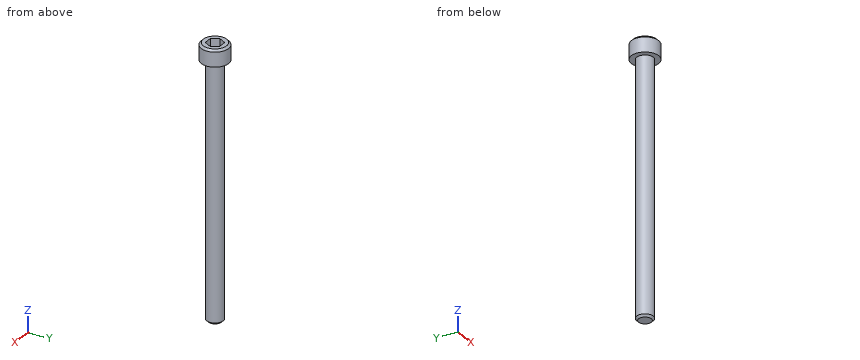
Autodesk Inventor part; units mm, degrees
ref_plane "YZ Plane" through (0, 0, 0) normal (1, 0, 0) x (0, 1, 0)
ref_plane "XZ Plane" through (0, 0, 0) normal (0, 1, 0) x (-1, 0, 0)
ref_plane "XY Plane" through (0, 0, 0) normal (0, 0, 1) x (1, 0, 0)
sketch "Sketch1" plane through (0, 0, 0) normal (0, 0, 1) x (1, 0, 0)
  circle A0 centre (0, 0) radius 3.429
  dimension "d0" = 6.858
extrude "Extrusion1" add sketch "Sketch1" along normal blind 4.1656
sketch "Sketch2" plane through (0, 0, 0) normal (0, 0, -1) x (-1, 0, 0)
  circle A0 centre (0, 0) radius 3.429
  circle A1 centre (0, 0) radius 2.0828
  dimension "d3" = 4.1656
extrude "Extrusion2" add sketch "Sketch2" along normal blind 63.5 contours A1
sketch "Sketch3" plane through (0, 0, 4.1656) normal (0, 0, 1) x (1, 0, 0)
  circle A0 centre (0, 0) radius 3.429
  line L0 (-1.0311, 1.7859) -> (1.0311, 1.7859)
  line L1 (1.0311, 1.7859) -> (2.0622, 0)
  line L2 (2.0622, 0) -> (1.0311, -1.7859)
  line L3 (1.0311, -1.7859) -> (-1.0311, -1.7859)
  line L4 (-1.0311, -1.7859) -> (-2.0622, 0)
  line L5 (-2.0622, 0) -> (-1.0311, 1.7859)
  dimension "d6" = 3.5719
extrude "Extrusion3" cut sketch "Sketch3" against normal blind 2.032 contours L0 L1 L2 L3 L4 L5
thread "Thread1"
chamfer "Chamfer1" distance 0.508 angle 45 1 edges at (2.0828, 0, -63.5)
chamfer "Chamfer2" distance 0.508 angle 45 1 edges at (-3.429, 0, 4.1656)
properties part number "10-32 x1000" material "Steel"
Geometry check sheet. Reference: the model listing, model coordinates, mm. Coordinates: 2 decimals unless noted, no trailing zeros. Order: outer loops, then holes, each group sorted by start corner. A loop starts at its lowest first (then second) coordinate and runs counter-clockwise, first axis right, second up. Notation, with made-up numbers: M 64,37 L 85,37 A32 ccw 85,70 Z; hole C 52,-5 d1. An arc over 180 degrees is marked long. One line per question, with ' | ' between items. Start each with the question number.
Item 1: Cross-section at B-B on z = -40.5. Enter the section's corners in (x, y).
Item 2: Gauge pin test, flat ends, axial feed: pin 1 (1 mm diameter, centred on y = 2, z = -54, fed in from -X) (3 decimals); pin 2 (3 mm diameter, centred on x = -2, z = -9, fed in from +Y); pin 3 (2 mm diameter, centred on y = 2.5, z = -24, fed in from +X) (3 decimals). Record the tip position at first contact, or that the pin passes through.
Item 3: Material ranges on L1, parallel to Z at x = -2.5, y = -1; L2, parallel to Y at x = 0, z = -44; L3, parallel to Z at x = 0, y = -1.5, recorded low to high. Write a range as [from, to].
Item 4: Cross-section at A-A on x = 0. Enter the section's corners in (y, z).
Findings:
1) outline: C 0,0 d4.17
2) pin 1: stops at x = -1.445 | pin 2: stops at y = 2.02 | pin 3: stops at x = 1.445
3) L1: z = [0, 4.17] | L2: y = [-2.08, 2.08] | L3: z = [-63.5, 2.13]
4) outline: M -3.43,0 L -2.08,0 L -2.08,-62.99 L -1.57,-63.5 L 1.57,-63.5 L 2.08,-62.99 L 2.08,0 L 3.43,0 L 3.43,3.66 L 2.92,4.17 L 1.79,4.17 L 1.79,2.13 L -1.79,2.13 L -1.79,4.17 L -2.92,4.17 L -3.43,3.66 Z
